```python
from build123d import *

# Parameters (mm, degrees)
F0_W     = 35.433
F0_H     = 203.2
F0_R     = 1.8288
F0_R_2   = 1.35255
F0_W_2   = 19.558
F0_H_2   = 40.64
F1_DEPTH = 1.70942
F3_DEPTH = 146.677299
F4_R     = 3.175


with BuildPart() as f1:
    # F0 (on Top) → F1 (new body)
    with BuildSketch(Plane.XY):
        with Locations((0, -65.397299)):
            Rectangle(F0_W, F0_H)
        with Locations((-14.5415, -163.822299)):
            Circle(F0_R, mode=Mode.SUBTRACT)
        with Locations((14.5415, -163.822299)):
            Circle(F0_R, mode=Mode.SUBTRACT)
        with Locations((-14.5415, 33.027701)):
            Circle(F0_R_2, mode=Mode.SUBTRACT)
        Rectangle(F0_W_2, F0_H_2, mode=Mode.SUBTRACT)
        with Locations((14.5415, 33.027701)):
            Circle(F0_R_2, mode=Mode.SUBTRACT)
    extrude(amount=F1_DEPTH)

    # F2 (on face) → F3 (join, through all)
    with BuildSketch(Plane.XZ.offset(166.997299)):
        with BuildLine():
            ThreePointArc((-19.119216, -0.581024), (-18.475644, -0.151003), (-17.7165, 0))
            Line((-17.7165, 0), (-17.7165, 1.70942))
            ThreePointArc((-17.7165, 1.70942), (-19.129811, 1.428295), (-20.327958, 0.627718))
            Line((-20.327958, 0.627718), (-22.573023, -1.617346))
            Line((-22.573023, -1.617346), (-21.36428, -2.826088))
            Line((-21.36428, -2.826088), (-19.119216, -0.581024))
        make_face()
        with BuildLine():
            Line((17.7165, 1.70942), (17.7165, 0))
            ThreePointArc((17.7165, 0), (18.475644, -0.151003), (19.119216, -0.581024))
            Line((19.119216, -0.581024), (21.36428, -2.826088))
            Line((21.36428, -2.826088), (22.573023, -1.617346))
            Line((22.573023, -1.617346), (20.327958, 0.627718))
            ThreePointArc((20.327958, 0.627718), (19.129811, 1.428295), (17.7165, 1.70942))
        make_face()
    extrude(amount=-F3_DEPTH)

    # F4
    f4_edges = [f1.edges().sort_by_distance(p)[0] for p in [
        (17.7165, 36.202701, 0.85471),
        (-17.7165, 36.202701, 0.85471),
    ]]
    fillet(f4_edges, radius=F4_R)


solid = f1.part
```
The listing builds one solid part. Answer for the finished solid, in the listing's coordinates (mm). A direction names the side the tool comes from. Round coordinates to 2 decimals unless told otherwise and drop trailing zeros. Loops run counter-clockwise (first coordinate to the right, second up) from the corner with the lowest first, then second, coordinate; pieces in that order, holes last.
Q1. For a pull along Y with two mould halves and no side action, classify faces 1 (the face through (20, -20.32, -1)), 2 (the face through (13.19, -162.59, 0.84)), 3 (the face through (0, -64, 0)) as released by +Y, released by -Y, zero draft, split by the parting line, or undercut.
Q2. Find the intervals of material crossed by line 1 (Y direction, x = 0, z = 1.35); line 2 (Y direction, x = -14.5, z = 0.3); line 3 (X direction, y = 16, z = 0.9), in increasing order.
Q3. Section A-A, the plane x = 7.5 is taken. Determine the outline of the cut face in (y, z).
Q4. Section C-C, the plane y = -81.5 is taken. Determine the outline of the cut face in (x, z), then the cut area to 3 significant figures.
Q5. Section B-B, the plane y = 16.5 is taken. Determine the outline of the cut face in (x, z), then the cut area to 3 significant figures.
Q6. Which of the six approach directions +Z, -Z, +X, -X, +Y, -Y give full straight-line access (tool end or side, diameter ignored) to faces 4 (the face through (-14.78, -162.01, 0.84)), 5 (the face through (-20, -20.32, -1))?
Q7. Given pin 1 Ø1.4 at (x, z) = (-19, -1) entering from +Y; pin 2 Ø5 at (x, y) = (14.54, -163.82) entering from -Z; pin 3 Ø2 at (y, z) = (-105, -0.5) entering from -X, each flat-ended and moving along its own axis, determine where each tip first touches the part or whether it passes through.
Completed:
1. face 1: released by +Y
1. face 2: undercut
1. face 3: zero draft
2. line 1: y = -167 to -20.32, 20.32 to 36.2
2. line 2: y = -167 to -165.65, -161.99 to 31.68, 34.38 to 36.2
2. line 3: x = -17.72 to -9.78, 9.78 to 17.72
3. outline: (-167, 0) - (-20.32, 0) - (-20.32, 1.71) - (-167, 1.71) - close; (20.32, 0) - (36.2, 0) - (36.2, 1.71) - (20.32, 1.71) - close
4. outline: (-22.57, -1.62) - (-21.36, -2.83) - (-19.12, -0.58) arc R1.98 cw to (-17.72, 0) - (17.72, 0) arc R1.98 cw to (19.12, -0.58) - (21.36, -2.83) - (22.57, -1.62) - (20.33, 0.63) arc R3.69 ccw to (17.72, 1.71) - (-17.72, 1.71) arc R3.69 ccw to (-20.33, 0.63) - close
4. area: 79.0 mm2
5. outline: (-17.72, 0) - (-9.78, 0) - (-9.78, 1.71) - (-17.72, 1.71) - close; (9.78, 0) - (17.72, 0) - (17.72, 1.71) - (9.78, 1.71) - close
5. area: 27.1 mm2
6. face 4: +Z, -Z
6. face 5: +Z, -Z, -X, +Y
7. pin 1: stops at y = -20.32
7. pin 2: stops at z = 0
7. pin 3: stops at x = -22.46
